```python
from build123d import *

# Parameters (mm, degrees)
F0_W     = 25.4
F0_H     = 25.4
F1_DEPTH = 12.7
F2_W     = 25.4
F2_H     = 25.4
F3_DEPTH = 25.4
F4_W     = 25.4
F4_H     = 25.4
F5_DEPTH = 25.4
F6_W     = 25.4
F6_H     = 25.4
F7_DEPTH = 25.4
F8_W     = 25.4
F8_H     = 25.4
F9_DEPTH = 25.4


with BuildPart() as f1:
    # F0 (on Front) → F1 (new body, symmetric)
    with BuildSketch(Plane.XZ):
        with Locations((12.7, 12.7)):
            Rectangle(F0_W, F0_H)
    extrude(amount=F1_DEPTH, both=True)

    # F2 (on face) → F3 (join)
    with BuildSketch(Plane(origin=(0, 0, 0), x_dir=(1, 0, 0), z_dir=(0, 0, -1))):
        with Locations((12.7, 0)):
            Rectangle(F2_W, F2_H)
    extrude(amount=F3_DEPTH)

    # F4 (on face) → F5 (join)
    with BuildSketch(Plane.YZ.offset(25.4)):
        with Locations((0, 12.7)):
            Rectangle(F4_W, F4_H)
    extrude(amount=F5_DEPTH)

    # F6 (on face) → F7 (join)
    with BuildSketch(Plane(origin=(0, 0, 0), x_dir=(0, -1, 0), z_dir=(-1, 0, 0))):
        with Locations((0, 12.7)):
            Rectangle(F6_W, F6_H)
    extrude(amount=F7_DEPTH)

    # F8 (on face) → F9 (join)
    with BuildSketch(Plane.XY.offset(25.4)):
        with Locations((12.7, 0)):
            Rectangle(F8_W, F8_H)
    extrude(amount=F9_DEPTH)


solid = f1.part
```
Work out the finished part from the listing and answer in its coordinate system (mm). A direction names the side the tool comes from. Coordinates: 2 decimals unless noted, no trailing zeros. Loops run counter-clockwise (first coordinate to the right, second up) from the corner with the lowest first, then second, coordinate; pieces in that order, holes last.
1) For faces 1 (the flat face through (25.4, 0, 38)), 2 (the flat face through (-13, 0, 0)), 3 (the flat face through (-13, 0, 25.4)), determine the directions among +Z, -Z, +X, -X, +Y, -Y from which every point of the face is accessible in a straight line to the end or side of a thin tool.
Results:
face 1: +Z, +X, +Y, -Y
face 2: -Z, -X, +Y, -Y
face 3: +Z, -X, +Y, -Y
2) Section A-A (y = 1.25) is taken. Give the vertices of the cut face in (x, z).
Results:
outline: (-25.4, 0) - (0, 0) - (0, -25.4) - (25.4, -25.4) - (25.4, 0) - (50.8, 0) - (50.8, 25.4) - (25.4, 25.4) - (25.4, 50.8) - (0, 50.8) - (0, 25.4) - (-25.4, 25.4) - close
3) Section C-C (x = 31.5) is taken. Give the vertices of the cut face in (y, z), plus the area to 3 significant figures.
Results:
outline: (-12.7, 0) - (12.7, 0) - (12.7, 25.4) - (-12.7, 25.4) - close
area: 645 mm2
4) Section B-B (z = 34) is taken. Give the vertices of the cut face in (x, y).
Results:
outline: (0, -12.7) - (25.4, -12.7) - (25.4, 12.7) - (0, 12.7) - close
5) Consider probe 1 along X at (y, z) = (-9.5, -5.5). Determine where the line is inside the solid, lowest interval first.
Results:
probe 1: x = 0 to 25.4
6) Flat-ended cylindrical pins translate along their axes: pin 1 (12.5 mm diameter, centred on y = -2.5, z = -8.5, fed in from +X); pin 2 (1.5 mm diameter, centred on x = 38.5, y = -5, fed in from -Z); pin 3 (6 mm diameter, centred on x = -7.5, y = 5, fed in from +Z). Find the tip coordinate at first contact, or state that the pin passes through.
Results:
pin 1: stops at x = 25.4
pin 2: stops at z = 0
pin 3: stops at z = 25.4
